Verification items for the finished model (mm, model axes). A direction names the side the tool comes from. Coordinates: 2 decimals unless noted, no trailing zeros. Write each loop counter-clockwise with the first axis right and the second up, starting at its lowest first coordinate (ties: lowest second). Pieces come first, ordered by that corner, then holes. Notation, with made-up numbers: (67.5, 6.25) -> (74.5, 6.25) arc R25 cw to (74.5, 38.25) -> close; hole circle Ø5 at (58.5, 17.25). An arc over 180 degrees is marked (long way). Write each question's results on one line, items separated by ' | '. Start each with the question number.
from build123d import *

# Parameters (mm, degrees)
SKETCH1_W           = 249.6
SKETCH1_H           = 267.4
SKETCH1_R           = 2.5
SKETCH1_W_2         = 33
SKETCH1_H_2         = 90
BOSS_EXTRUDE1_DEPTH = 5
SKETCH6_W           = 249.6
SKETCH6_H           = 131.304588604
CUT_EXTRUDE4_DEPTH  = 6


with BuildPart() as part:
    # Sketch1 → Boss-Extrude1 (new body)
    with BuildSketch(Plane.XY):
        with Locations((124.8, -202.7)):
            Rectangle(SKETCH1_W, SKETCH1_H)
        with Locations((245.6, -193.5)):
            Circle(SKETCH1_R, mode=Mode.SUBTRACT)
        with Locations((245.6, -244.5)):
            Circle(SKETCH1_R, mode=Mode.SUBTRACT)
        with Locations((4, -244.5)):
            Circle(SKETCH1_R, mode=Mode.SUBTRACT)
        with Locations((4, -193.5)):
            Circle(SKETCH1_R, mode=Mode.SUBTRACT)
        with Locations((201.66, -219)):
            Rectangle(SKETCH1_W_2, SKETCH1_H_2, mode=Mode.SUBTRACT)
        with Locations((47.94, -219)):
            Rectangle(SKETCH1_W_2, SKETCH1_H_2, mode=Mode.SUBTRACT)
    extrude(amount=BOSS_EXTRUDE1_DEPTH)

    # Sketch6 → Cut-Extrude4 (cut, through all)
    with BuildSketch(Plane.XY.offset(5)):
        with BuildLine():
            Line((43.402860001, -44), (0, -44))
            Line((0, -44), (0, -169))
            Line((0, -169), (43.402860001, -169))
            ThreePointArc((43.402860001, -169), (105.902860001, -106.5), (43.402860001, -44))
        make_face()
        with BuildLine():
            Line((206.197139999, -169), (249.6, -169))
            Line((249.6, -169), (249.6, -44))
            Line((249.6, -44), (206.197139999, -44))
            ThreePointArc((206.197139999, -44), (143.697139999, -106.5), (206.197139999, -169))
        make_face()
        with Locations((124.8, -270.747705698)):
            Rectangle(SKETCH6_W, SKETCH6_H)
    extrude(amount=-CUT_EXTRUDE4_DEPTH, mode=Mode.SUBTRACT)


solid = part.part
1. Tool access check on faces 5 (the flat face through (124, -157, 5)), 6 (the cylindrical face through (4, -191, 2)), 7 (the flat face through (21, -169, 3)), 8 (the flat face through (48, -174, 2)), 9 (the flat face through (228, -169, 3)). Record the directions out of +Z, -Z, +X, -X, +Y, -Y that give a thin tool (end or side, any length) a straight path to the whole face; none if there is none.
2. Sectioned sample at D-D on x = 230.5. Record the cut outline in (y, z).
3. Depth check by flat-ended pin: pin 1 Ø2 at (y, z) = (-143.5, 2.5) entering from +X; pin 2 Ø2.5 at (x, z) = (205.5, 2.5) entering from -Y; pin 3 Ø2.5 at (x, z) = (220, 2) entering from +Y. Enter the tip coordinate at first touch or a pass-through.
4. Sectioned sample at B-B on x = 4. Record the cut outline in (y, z).
5. Sectioned sample at C-C on y = -193.5. Record the cut outline in (x, z).
6. Mould release check, pull along X, two halves, no side actions. Record for faces 1 (the flat face through (201, -174, 2)), 2 (the flat face through (0, -187, 2)), 3 (the flat face through (64.44, -190, 2)), 4 (the flat face through (249.6, -187, 2)): +X half, -X half, draft (parallel to the pull), parting line (faces both ways), or undercut.
7. Material ranges on probe 1 along X at (y, z) = (-174.5, 3.75); probe 2 along X at (y, z) = (-193.5, 2.15); probe 3 along Y at (x, z) = (245.6, 2.85), recorded low to high. Write a range as from..to.
8. Sectioned sample at A-A on z = 2.45. Record the cut outline in (x, y).
Computed values:
1) face 5: +Z, +X, -X, +Y, -Y | face 6: +Z, -Z | face 7: +Z, -Z, -X, +Y | face 8: +Z, -Z, -Y | face 9: +Z, -Z, +X, +Y
2) outline: (-205.1, 0) -> (-169, 0) -> (-169, 5) -> (-205.1, 5) -> close
3) pin 1: stops at x = 156.58 | pin 2: stops at y = -174 | pin 3: stops at y = -169
4) outline: (-205.1, 0) -> (-196, 0) -> (-196, 5) -> (-205.1, 5) -> close; (-191, 0) -> (-169, 0) -> (-169, 5) -> (-191, 5) -> close
5) outline: (0, 0) -> (1.5, 0) -> (1.5, 5) -> (0, 5) -> close; (6.5, 0) -> (31.44, 0) -> (31.44, 5) -> (6.5, 5) -> close; (64.44, 0) -> (185.16, 0) -> (185.16, 5) -> (64.44, 5) -> close; (218.16, 0) -> (243.1, 0) -> (243.1, 5) -> (218.16, 5) -> close; (248.1, 0) -> (249.6, 0) -> (249.6, 5) -> (248.1, 5) -> close
6) face 1: undercut | face 2: -X half | face 3: undercut | face 4: +X half
7) probe 1: x = 0..31.44, 64.44..185.16, 218.16..249.6 | probe 2: x = 0..1.5, 6.5..31.44, 64.44..185.16, 218.16..243.1, 248.1..249.6 | probe 3: y = -205.1..-196, -191..-169
8) outline: (0, -205.1) -> (31.44, -205.1) -> (31.44, -174) -> (64.44, -174) -> (64.44, -205.1) -> (185.16, -205.1) -> (185.16, -174) -> (218.16, -174) -> (218.16, -205.1) -> (249.6, -205.1) -> (249.6, -169) -> (206.2, -169) arc R62.5 cw to (156.2, -69) -> (93.4, -69) arc R62.5 cw to (43.4, -169) -> (0, -169) -> close; hole circle Ø5 at (4, -193.5); hole circle Ø5 at (245.6, -193.5)
